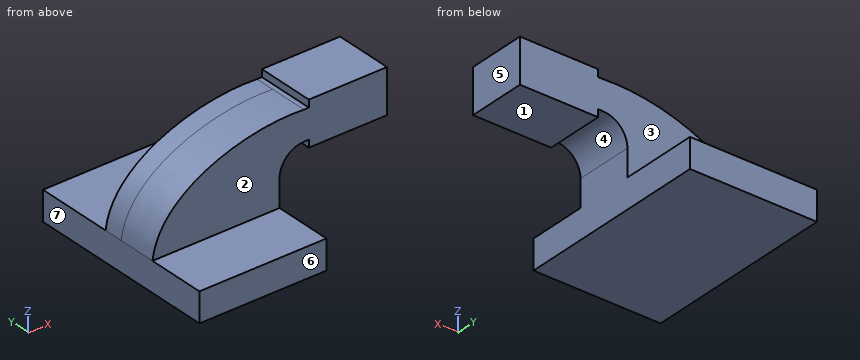
```python
from build123d import *

# Parameters (mm, degrees)
F1_DEPTH = 63.5
F2_DEPTH = 25.4
F3_DEPTH = 12.7


with BuildPart() as f1:
    # F0 (on Front) → F1 (new body, symmetric)
    with BuildSketch(Plane.XZ):
        Polygon((22.225, 9.525), (-41.275, 9.525), (-41.275, -9.525), (41.275, -9.525), (41.275, 9.525), align=None)
    extrude(amount=F1_DEPTH, both=True)

    # F0 (on Front) → F2 (join)
    with BuildSketch(Plane.XZ):
        with BuildLine():
            add(Edge.make_bspline(
                [(-41.275, 9.525), (-36.934671, 47.172504), (18.990146, 64.688085), (57.15, 61.9252)],
                knots=[0, 0, 0, 0, 111.504536, 111.504536, 111.504536, 111.504536], degree=3))
            Line((-41.275, 9.525), (22.225, 9.525))
            Line((22.225, 9.525), (22.225, 27.0002))
            ThreePointArc((22.225, 27.0002), (32.454296, 51.695904), (57.15, 61.9252))
        make_face()
        Polygon((22.225, 9.525), (-41.275, 9.525), (-41.275, -9.525), (41.275, -9.525), (41.275, 9.525), align=None)
        with BuildLine():
            Line((22.225, 27.0002), (22.225, 9.525))
            Line((22.225, 9.525), (41.275, 9.525))
            Line((41.275, 9.525), (41.275, 27.0002))
            ThreePointArc((41.275, 27.0002), (45.92468, 38.22552), (57.15, 42.8752))
            Line((57.15, 42.8752), (60.325, 42.8752))
            Line((60.325, 42.8752), (60.325, 61.9252))
            Line((60.325, 61.9252), (57.15, 61.9252))
            ThreePointArc((57.15, 61.9252), (32.454296, 51.695904), (22.225, 27.0002))
        make_face()
        Polygon((60.325, 66.675), (60.325, 61.9252), (60.325, 42.8752), (60.325, 38.1), (111.125, 38.1), (111.125, 66.675), align=None)
    extrude(amount=F2_DEPTH)

    # F0 (on Front) → F3 (join, symmetric)
    with BuildSketch(Plane.XZ):
        with BuildLine():
            add(Edge.make_bspline(
                [(-41.275, 9.525), (-36.934671, 47.172504), (18.990146, 64.688085), (57.15, 61.9252)],
                knots=[0, 0, 0, 0, 111.504536, 111.504536, 111.504536, 111.504536], degree=3))
            Line((-41.275, 9.525), (22.225, 9.525))
            Line((22.225, 9.525), (22.225, 27.0002))
            ThreePointArc((22.225, 27.0002), (32.454296, 51.695904), (57.15, 61.9252))
        make_face()
        Polygon((22.225, 9.525), (-41.275, 9.525), (-41.275, -9.525), (41.275, -9.525), (41.275, 9.525), align=None)
        with BuildLine():
            Line((22.225, 27.0002), (22.225, 9.525))
            Line((22.225, 9.525), (41.275, 9.525))
            Line((41.275, 9.525), (41.275, 27.0002))
            ThreePointArc((41.275, 27.0002), (45.92468, 38.22552), (57.15, 42.8752))
            Line((57.15, 42.8752), (60.325, 42.8752))
            Line((60.325, 42.8752), (60.325, 61.9252))
            Line((60.325, 61.9252), (57.15, 61.9252))
            ThreePointArc((57.15, 61.9252), (32.454296, 51.695904), (22.225, 27.0002))
        make_face()
        Polygon((60.325, 66.675), (60.325, 61.9252), (60.325, 42.8752), (60.325, 38.1), (111.125, 38.1), (111.125, 66.675), align=None)
    extrude(amount=F3_DEPTH, both=True)


solid = f1.part
```
The listing builds one solid part. Answer for the finished solid, in the listing's coordinates (mm). Face numbers are marked on the shaded views. A direction names the side the tool comes from. Round coordinates to 2 decimals unless told otherwise and drop trailing zeros. Order: outer loops, then holes, each group sorted by start corner. A loop starts at its lowest first (then second) coordinate and runs counter-clockwise, first axis right, second up. Notation, with made-up numbers: (30.25, 50.5) - (75.25, 50.5) arc R19 ccw to (75.25, 58.5) - close; hole circle Ø5 at (47, 34). An arc over 180 degrees is marked (long way). Put each result on its own line as item: value. Start each with the question number.
(1) Straight lines are drawn through the part: probe 1 along Z at (x, y) = (85.5, 10) (3 decimals); probe 2 along Z at (x, y) = (4.5, -54) (3 decimals); probe 3 along Y at (x, z) = (26, 52). For each, find the intervals that lie inside material, in ascending order. Write a range as from..to.
(2) Given P1, Ø17, axis at x = 63.5, z = 24.5, coming from the +Y side; P2, Ø2, axis at x = 15.5, z = 15.5, coming from the +Y side; P3, Ø2.5, axis at y = -12.5, z = 64.5, coming from the -X side (3 decimals); P4, Ø1.6, axis at x = 59, y = -14, coming from the -Z side, each flat-ended and moving along its own axis, determine where each tip first touches the part or whether it passes through.
(3) For the marked faces 1, 2 and 3, determine the directions among +Z, -Z, +X, -X, +Y, -Y from which every point of the face is accessible in a straight line to the end or side of a thin tool.
(4) Find section B-B (x = 77). Give the vertices of the cut face in (y, z) (3 decimals).
(5) Find section A-A (y = 28). Give the vertices of the cut face in (x, z) (3 decimals).
(6) Determine the mould class of the marked faces 4, 5, 6 and 7 for opening direction X: released by +X, released by -X, zero draft, split by the parting line, or undercut.
Reply:
1. probe 1: 38.1..66.675
1. probe 2: -9.525..9.525
1. probe 3: -25.4..12.7
2. P1: through
2. P2: y = 12.7
2. P3: x = 60.325
2. P4: z = 42.88
3. face 1: -Z, +X, +Y, -Y
3. face 2: +Z, +X, -X, -Y
3. face 3: +Z, +X, -X, +Y
4. outline: (-25.4, 38.1) - (12.7, 38.1) - (12.7, 66.675) - (-25.4, 66.675) - close
5. outline: (-41.275, -9.525) - (41.275, -9.525) - (41.275, 9.525) - (-41.275, 9.525) - close
6. face 4: undercut
6. face 5: released by +X
6. face 6: zero draft
6. face 7: released by -X
